from build123d import *

# Parameters (mm, degrees)
SKETCH_1_R      = 5
SKETCH_1_R_2    = 1.35
EXTRUDE_1_DEPTH = 3


with BuildPart() as part:
    # 草图1 → 凸台-拉伸1 (new body)
    with BuildSketch(Plane(origin=(0, 0, 0), x_dir=(1, 0, 0), z_dir=(0, 1, 0))):
        with BuildLine():
            Line((14.282856857, -14), (140, -14))
            ThreePointArc((140, -14), (154, 0), (140, 14))
            Line((140, 14), (14.282856857, 14))
            ThreePointArc((14.282856857, 14), (-20, 0), (14.282856857, -14))
        make_face()
        with Locations(Location((140, 0, 0), (0, 0, 270))):
            Circle(SKETCH_1_R, mode=Mode.SUBTRACT)
        with Locations(Location((140, 11, 0), (0, 0, 270))):
            Circle(SKETCH_1_R_2, mode=Mode.SUBTRACT)
        with Locations(Location((147.778174593, 7.778174593, 0), (0, 0, 270))):
            Circle(SKETCH_1_R_2, mode=Mode.SUBTRACT)
        with Locations(Location((151, 0, 0), (0, 0, 270))):
            Circle(SKETCH_1_R_2, mode=Mode.SUBTRACT)
        with Locations(Location((147.778174593, -7.778174593, 0), (0, 0, 270))):
            Circle(SKETCH_1_R_2, mode=Mode.SUBTRACT)
        with Locations(Location((140, -11, 0), (0, 0, 270))):
            Circle(SKETCH_1_R_2, mode=Mode.SUBTRACT)
        with Locations(Location((132.221825407, -7.778174593, 0), (0, 0, 270))):
            Circle(SKETCH_1_R_2, mode=Mode.SUBTRACT)
        with Locations(Location((129, 0, 0), (0, 0, 270))):
            Circle(SKETCH_1_R_2, mode=Mode.SUBTRACT)
        with Locations(Location((132.221825407, 7.778174593, 0), (0, 0, 270))):
            Circle(SKETCH_1_R_2, mode=Mode.SUBTRACT)
    extrude(amount=EXTRUDE_1_DEPTH)


solid = part.part
Geometry check sheet. Reference: the model listing, model coordinates, mm. A direction names the side the tool comes from. Give positions to 0.01 mm unless a question says otherwise; leave off trailing zeros. Order: outer loops, then holes, each group sorted by start corner. A loop starts at its lowest first (then second) coordinate and runs counter-clockwise, first axis right, second up. Notation, with made-up numbers: M 43.5,13.25 L 76.5,13.25 A29 ccw 76.5,45.25 Z; hole C 85.5,66 d5. An arc over 180 degrees is marked long. Use a Markdown table: item, result.
Item 1: Draft check along Z on faces 1 (the flat face through (66, 3, 0)), 2 (the cylindrical face through (146.46, 1.48, -8.07)), 3 (the cylindrical face through (154, 1, 0)). Enter one of: +Z half, -Z half, draft (parallel to the pull), parting line (faces both ways), or undercut.
Answers follow:
| item | result |
|---|---|
| face 1 | draft |
| face 2 | undercut |
| face 3 | parting line |
Item 2: Tool access check on faces 4 (the flat face through (76, 1, 14)), 5 (the flat face through (78, 1, -14)), 6 (the cylindrical face through (132.28, 1.48, 6.43)). Record the directions out of +Z, -Z, +X, -X, +Y, -Y that give a thin tool (end or side, any length) a straight path to the whole face; none if there is none.
Answers follow:
| item | result |
|---|---|
| face 4 | +Z, +X, +Y, -Y |
| face 5 | -Z, +X, +Y, -Y |
| face 6 | +Y, -Y |
Item 3: Section check A-A (z = -3.5). Record the cut outline in (x, y), and give its area (3 significant figures).
Answers follow:
| item | result |
|---|---|
| outline | M -19.69,0 L 136.43,0 L 136.43,3 L -19.69,3 Z; M 143.57,0 L 153.56,0 L 153.56,3 L 143.57,3 Z |
| area | 498 mm2 |
Item 4: Section check C-C (x = 125.5). Record the cut outline in (y, z), and give its area (3 significant figures).
Answers follow:
| item | result |
|---|---|
| outline | M 0,-14 L 3,-14 L 3,14 L 0,14 Z |
| area | 84.0 mm2 |
Item 5: Depth check by flat-ended pin: P1, Ø5, axis at x = 79.5, z = -8, coming from the -Y side; P2, Ø1.6, axis at x = 147.78, z = -7.78, coming from the -Y side; P3, Ø0.9, axis at x = 52, y = 1.5, coming from the +Z side; P4, Ø0.9, axis at x = 56.5, y = 1.5, coming from the -Z side. Enter the tip coordinate at first touch or a pass-through.
Answers follow:
| item | result |
|---|---|
| P1 | stops at y = 0 |
| P2 | passes through |
| P3 | stops at z = 14 |
| P4 | stops at z = -14 |
Item 6: Material ranges on line 1 along X through (y, z) = (1.4, 8); line 2 along Z through (x, y) = (105, 0.8); line 3 along X through (y, z) = (2.3, 1.5), recorded low to high.
Answers follow:
| item | result |
|---|---|
| line 1 | x = -18.33 to 130.89, 133.55 to 146.45, 149.11 to 151.49 |
| line 2 | z = -14 to 14 |
| line 3 | x = -19.94 to 135.23, 144.77 to 153.92 |
Item 7: Section check B-B (y = 0.9). State how many separate pieces and enclosed holes the cut face has, and give its area (3 significant figures).
Answers follow:
| item | result |
|---|---|
| separate pieces | 1 |
| enclosed holes | 9 |
| area | 4,850 mm2 |
